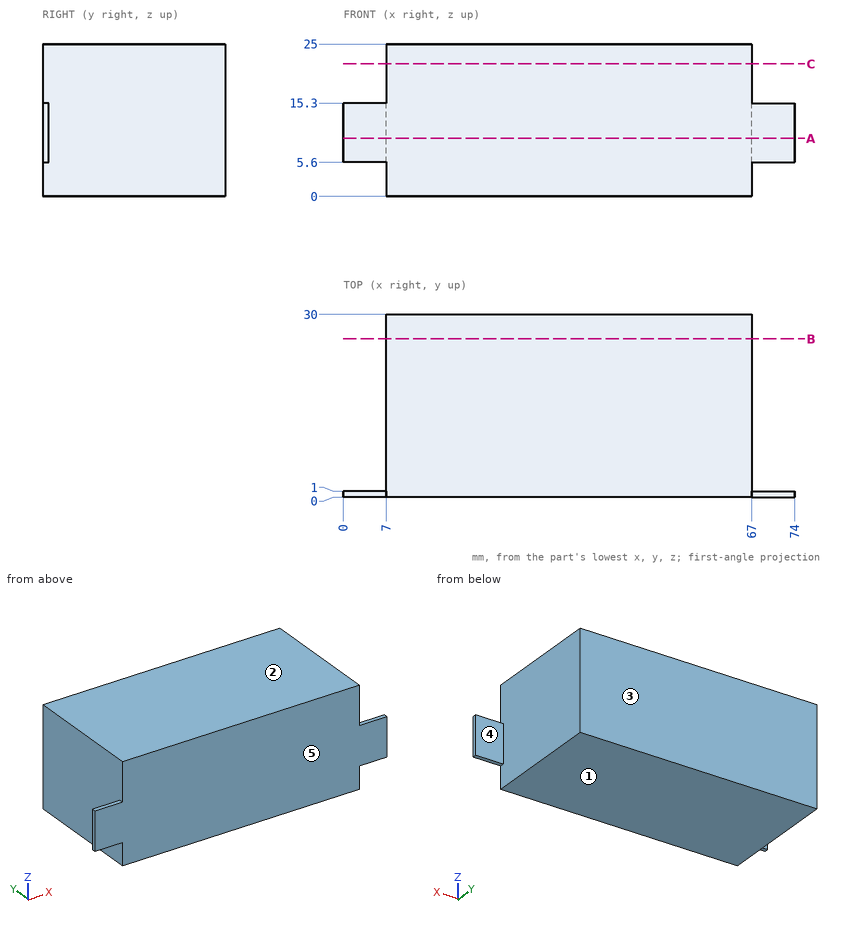
Answer from the drawing. Dimensions are ordinates in mm from the lowest x, y and z of the part. A direction names the side the tool comes from. Coordinates: 2 decimals unless noted, no trailing zeros. Order: outer loops, then holes, each group sorted by start corner. A loop starts at its lowest first (then second) coordinate and runs counter-clockwise, first axis right, second up. Notation, with made-up numbers: (12.25, 49.25) - (28.25, 49.25) arc R33 cw to (28.25, 82.25) - close; hole circle Ø11 at (83.5, 71.5). An arc over 180 degrees is marked (long way). Answer as a JSON object with one key per item and string values. Group by question number.
Item 1: Section B-B (y = 26) is taken. Give the vertices of the cut face in (x, z).
Item 2: Section A-A (z = 9.5) is taken. Give the vertices of the cut face in (x, y), plus the area to 3 significant figures.
Item 3: Section C-C (z = 21.75) is taken. Give the vertices of the cut face in (x, y).
Item 4: The mould has two halves that part along Z. Classify the marked faces 1, 2 and 3: +Z half, -Z half, draft (parallel to the pull), parting line (faces both ways), or undercut.
Item 5: Flat-ended cylindrical pins translate along their axes: P1, Ø3, axis at y = 12.5, z = 15.5, coming from the -X side; P2, Ø1, axis at y = 25.5, z = 9, coming from the +X side; P3, Ø2, axis at x = 71.5, z = 9, coming from the +Y side. Find the tip coordinate at first contact, or state that the pin passes through.
Item 6: Consider probe 1 along X at (y, z) = (4.5, 13.25). Determine where the line is inside the solid, lowest interval first. Write a range as from..to.
Item 7: A tool of negligible diameter and unlimited length cuts with its end or side. For the marked faces 4 and 5, from which of +Z, -Z, +X, -X, +Y, -Y can it reach the whole face along a straight path? Write none if from no direction.
Results are:
{
 "1": {"outline": "(7, 0) - (67, 0) - (67, 25) - (7, 25) - close"},
 "2": {"outline": "(0, 0) - (74, 0) - (74, 1) - (67, 1) - (67, 30) - (7, 30) - (7, 1) - (0, 1) - close", "area": "1,810 mm^2"},
 "3": {"outline": "(7, 0) - (67, 0) - (67, 30) - (7, 30) - close"},
 "4": {"face 1": "-Z half", "face 2": "+Z half", "face 3": "draft"},
 "5": {"P1": "stops at x = 7", "P2": "stops at x = 67", "P3": "stops at y = 1"},
 "6": {"probe 1": "x = 7..67"},
 "7": {"face 4": "+Z, -Z, +X, +Y", "face 5": "+Z, -Z, +X, -X, -Y"}
}
